The listing builds one solid part. Answer for the finished solid, in the listing's coordinates (mm). A direction names the side the tool comes from. Give positions to 0.01 mm unless a question says otherwise; leave off trailing zeros. Order: outer loops, then holes, each group sorted by start corner. A loop starts at its lowest first (then second) coordinate and runs counter-clockwise, first axis right, second up. Notation, with made-up numbers: (88.5, 15) - (108.5, 15) arc R29 cw to (108.5, 38) - close; hole circle Ø5 at (85, 14). An arc over 180 degrees is marked (long way). Answer in a Markdown table with one row per item.
from build123d import *

# Parameters (mm, degrees)
ESQUISSE2_R             = 3.1
ENL_V_MAT_EXTRU_1_DEPTH = 21
ESQUISSE4_OUTSIDE_W     = 168.986
ESQUISSE4_OUTSIDE_H     = 168.986
ESQUISSE4_OUTSIDE_R     = 42.05
ENL_V_MAT_EXTRU_3_DEPTH = 4
ESQUISSE3_R             = 5.1
ENL_V_MAT_EXTRU_2_DEPTH = 6.2
ENL_V_MAT_EXTRU_4_DEPTH = 6.2
CONG_2_R                = 2


with BuildPart() as part:
    # Esquisse1 → Révolution1 (revolve)
    with BuildSketch(Plane.XY):
        Polygon((-34.05, 0), (-34.05, 15), (-29.05, 15), (-29.05, 20), (-47.1, 20), (-47.1, 14), (-50.3, 14), (-50.3, 20), (-65, 20), (-65, 0), align=None)
    revolve(axis=Axis((0, 0, 0), (0, 1, 0)))

    # Esquisse2 → Enlèv. mat.-Extru.1 (cut, through all)
    with BuildSketch(Plane.XZ):
        with Locations((0, 58)):
            Circle(ESQUISSE2_R)
        with Locations((41.012193309, 41.012193309)):
            Circle(ESQUISSE2_R)
        with Locations((58, 0)):
            Circle(ESQUISSE2_R)
        with Locations((41.012193309, -41.012193309)):
            Circle(ESQUISSE2_R)
        with Locations((0, -58)):
            Circle(ESQUISSE2_R)
        with Locations((-41.012193309, -41.012193309)):
            Circle(ESQUISSE2_R)
        with Locations((-58, 0)):
            Circle(ESQUISSE2_R)
        with Locations((-41.012193309, 41.012193309)):
            Circle(ESQUISSE2_R)
    extrude(amount=-ENL_V_MAT_EXTRU_1_DEPTH, mode=Mode.SUBTRACT)

    # Esquisse4 outside → Enlèv. mat.-Extru.3 (cut)
    with BuildSketch(Plane.XZ):
        Rectangle(ESQUISSE4_OUTSIDE_W, ESQUISSE4_OUTSIDE_H)
        Circle(ESQUISSE4_OUTSIDE_R, mode=Mode.SUBTRACT)
    extrude(amount=-ENL_V_MAT_EXTRU_3_DEPTH, mode=Mode.SUBTRACT)

    # Esquisse3 → Enlèv. mat.-Extru.2 (cut)
    with BuildSketch(Plane.XZ.offset(-4)):
        with Locations((0, 58)):
            Circle(ESQUISSE3_R)
        with Locations((41.012193309, 41.012193309)):
            Circle(ESQUISSE3_R)
        with Locations((58, 0)):
            Circle(ESQUISSE3_R)
        with Locations((41.012193309, -41.012193309)):
            Circle(ESQUISSE3_R)
        with Locations((0, -58)):
            Circle(ESQUISSE3_R)
        with Locations((-41.012193309, -41.012193309)):
            Circle(ESQUISSE3_R)
        with Locations((-58, 0)):
            Circle(ESQUISSE3_R)
        with Locations((-41.012193309, 41.012193309)):
            Circle(ESQUISSE3_R)
    extrude(amount=-ENL_V_MAT_EXTRU_2_DEPTH, mode=Mode.SUBTRACT)

    # Esquisse5 → Enlèv. mat.-Extru.4 (cut)
    with BuildSketch(Plane.XZ.offset(-4)):
        with BuildLine():
            Line((5.2, -58), (5.2, -69.173010208))
            ThreePointArc((5.2, -69.173010208), (0, -74.373010208), (-5.2, -69.173010208))
            Line((-5.2, -69.173010208), (-5.2, -58))
            ThreePointArc((-5.2, -58), (0, -52.8), (5.2, -58))
        make_face()
        with BuildLine():
            Line((-37.335238047, -44.689148571), (-45.235749331, -52.589659855))
            ThreePointArc((-45.235749331, -52.589659855), (-52.589659855, -52.589659855), (-52.589659855, -45.235749331))
            Line((-52.589659855, -45.235749331), (-44.689148571, -37.335238047))
            ThreePointArc((-44.689148571, -37.335238047), (-37.335238047, -37.335238047), (-37.335238047, -44.689148571))
        make_face()
        with BuildLine():
            Line((-58, -5.2), (-69.173010208, -5.2))
            ThreePointArc((-69.173010208, -5.2), (-74.373010208, 0), (-69.173010208, 5.2))
            Line((-69.173010208, 5.2), (-58, 5.2))
            ThreePointArc((-58, 5.2), (-52.8, 0), (-58, -5.2))
        make_face()
        with BuildLine():
            Line((-44.689148571, 37.335238047), (-52.589659855, 45.235749331))
            ThreePointArc((-52.589659855, 45.235749331), (-52.589659855, 52.589659855), (-45.235749331, 52.589659855))
            Line((-45.235749331, 52.589659855), (-37.335238047, 44.689148571))
            ThreePointArc((-37.335238047, 44.689148571), (-37.335238047, 37.335238047), (-44.689148571, 37.335238047))
        make_face()
        with BuildLine():
            Line((-5.2, 58), (-5.2, 69.173010208))
            ThreePointArc((-5.2, 69.173010208), (0, 74.373010208), (5.2, 69.173010208))
            Line((5.2, 69.173010208), (5.2, 58))
            ThreePointArc((5.2, 58), (0, 52.8), (-5.2, 58))
        make_face()
        with BuildLine():
            Line((37.335238047, 44.689148571), (45.235749331, 52.589659855))
            ThreePointArc((45.235749331, 52.589659855), (52.589659855, 52.589659855), (52.589659855, 45.235749331))
            Line((52.589659855, 45.235749331), (44.689148571, 37.335238047))
            ThreePointArc((44.689148571, 37.335238047), (37.335238047, 37.335238047), (37.335238047, 44.689148571))
        make_face()
        with BuildLine():
            Line((58, 5.2), (69.173010208, 5.2))
            ThreePointArc((69.173010208, 5.2), (74.373010208, 0), (69.173010208, -5.2))
            Line((69.173010208, -5.2), (58, -5.2))
            ThreePointArc((58, -5.2), (52.8, 0), (58, 5.2))
        make_face()
        with BuildLine():
            Line((44.689148571, -37.335238047), (52.589659855, -45.235749331))
            ThreePointArc((52.589659855, -45.235749331), (52.589659855, -52.589659855), (45.235749331, -52.589659855))
            Line((45.235749331, -52.589659855), (37.335238047, -44.689148571))
            ThreePointArc((37.335238047, -44.689148571), (37.335238047, -37.335238047), (44.689148571, -37.335238047))
        make_face()
    extrude(amount=-ENL_V_MAT_EXTRU_4_DEPTH, mode=Mode.SUBTRACT)

    # Congé2
    cong_2_edges = [part.edges().sort_by_distance(p)[0] for p in [
        (49.491581748, 7.1, -42.137671223),
        (42.137671223, 7.1, -49.491581748),
        (64.791666131, 7.1, 5.2),
        (64.791666131, 7.1, -5.2),
        (42.137671223, 7.1, 49.491581748),
        (49.491581748, 7.1, 42.137671223),
        (-5.2, 7.1, 64.791666131),
        (5.2, 7.1, 64.791666131),
        (-49.491581748, 7.1, 42.137671223),
        (-42.137671223, 7.1, 49.491581748),
        (-64.791666131, 7.1, -5.2),
        (-64.791666131, 7.1, 5.2),
        (-42.137671223, 7.1, -49.491581748),
        (-49.491581748, 7.1, -42.137671223),
        (5.2, 7.1, -64.791666131),
        (-5.2, 7.1, -64.791666131),
    ]]
    fillet(cong_2_edges, radius=CONG_2_R)


solid = part.part
Item 1: Each of these flat-tipped pins is pushed along its axis until it touches: P1, Ø8, axis at x = 58, z = 0, coming from the -Y side; P2, Ø6, axis at x = 57.5, z = -3, coming from the -Y side; P3, Ø1.4, axis at y = 7.5, z = 60.5, coming from the -X side. Where does it stop, or does it pass through?
Answer block:
| item | result |
|---|---|
| P1 | y = 10.2 |
| P2 | y = 4 |
| P3 | x = -25.47 |
Item 2: Find section C-C on x = -9. Write down the section's boundary in (y, z), then the cut area to 3 significant figures.
Answer block:
| item | result |
|---|---|
| outline | (0, -41.08) - (4, -41.08) - (4, -64.37) - (20, -64.37) - (20, -49.49) - (14, -49.49) - (14, -46.23) - (20, -46.23) - (20, -27.62) - (15, -27.62) - (15, -32.84) - (0, -32.84) - close; (0, 32.84) - (15, 32.84) - (15, 27.62) - (20, 27.62) - (20, 46.23) - (14, 46.23) - (14, 49.49) - (20, 49.49) - (20, 64.37) - (4, 64.37) - (4, 41.08) - (0, 41.08) - close |
| area | 1,090 mm² |
Item 3: Which of the six approach directions +Z, -Z, +X, -X, +Y, -Y give full straight-line access (tool end or side, diameter ignored) to faces 1 (the face through (0, 10.2, -62)), 2 (the face through (15, 14, 45)), 3 (the face through (62, 10.2, 0)), 4 (the face through (-41.16, 7.06, 49.49))?
Answer block:
| item | result |
|---|---|
| face 1 | -Z, -Y |
| face 2 | +Y |
| face 3 | +X, -Y |
| face 4 | -X, -Y |
Item 4: Find section A-A on y = 17. Count the separate pieces of the cut face and the enclosed holes in it, then the cut area to 3 significant figures.
Answer block:
| item | result |
|---|---|
| separate pieces | 2 |
| enclosed holes | 10 |
| area | 9,400 mm² |
Item 5: Determine the mould class of faces 5 (the face through (-46.288, 7.057, 38.934)), 6 (the face through (37.255, 7.057, -37.417)), 7 (the face through (-0.1, 7.1, -52.8)), 8 (the face through (-33.369, 1.972, -25.587)) for opening direction Z: pulls with the +Z half, pulls with the -Z half, needs draft (parallel to the pull), parting line crosses it, or undercut.
Answer block:
| item | result |
|---|---|
| face 5 | pulls with the +Z half |
| face 6 | undercut |
| face 7 | pulls with the -Z half |
| face 8 | parting line crosses it |
Item 6: Consider line 1 (Z direction, x = 0, y = 17.9); line 2 (Z direction, x = -18, y = 18.25); line 3 (Z direction, x = 14, y = 14.5). Determine where each line is inside the solid, lowest interval first.
Answer block:
| item | result |
|---|---|
| line 1 | -65 to -61.1, -54.9 to -50.3, -47.1 to -29.05, 29.05 to 47.1, 50.3 to 54.9, 61.1 to 65 |
| line 2 | -62.46 to -46.97, -43.52 to -22.8, 22.8 to 43.52, 46.97 to 62.46 |
| line 3 | -63.47 to -48.31, -44.97 to -31.04, 31.04 to 44.97, 48.31 to 63.47 |
Item 7: Find section B-B on z = 26.5. Write down the section's boundary in (x, y), then the cut area to 3 significant figures.
Answer block:
| item | result |
|---|---|
| outline | (-59.35, 4) - (-32.65, 4) - (-32.65, 0) - (-21.38, 0) - (-21.38, 15) - (-11.9, 15) - (-11.9, 20) - (-38.94, 20) - (-38.94, 14) - (-42.75, 14) - (-42.75, 20) - (-59.35, 20) - close; (11.9, 15) - (21.38, 15) - (21.38, 0) - (32.65, 0) - (32.65, 4) - (59.35, 4) - (59.35, 20) - (42.75, 20) - (42.75, 14) - (38.94, 14) - (38.94, 20) - (11.9, 20) - close |
| area | 1,350 mm² |
Item 8: Find section D-D on z = -31.5. Write down the section's boundary in (x, y).
Answer block:
| item | result |
|---|---|
| outline | (-56.86, 4) - (-27.86, 4) - (-27.86, 0) - (-12.93, 0) - (-12.93, 15) - (12.93, 15) - (12.93, 0) - (27.86, 0) - (27.86, 4) - (56.86, 4) - (56.86, 20) - (39.22, 20) - (39.22, 14) - (35.02, 14) - (35.02, 20) - (-35.02, 20) - (-35.02, 14) - (-39.22, 14) - (-39.22, 20) - (-56.86, 20) - close |
